Can you work these out from the model? Positions are in its coordinate system, mm. Face numbers are marked on the shaded views. A direction names the side the tool comes from. Round coordinates to 2 decimals unless told otherwise and drop trailing zeros. Loops run counter-clockwise (first coordinate to the right, second up) from the corner with the lowest first, then second, coordinate; pieces in that order, holes last. Notation, with made-up numbers: (79.25, -4.75) -> (102.25, -4.75) arc R26 ccw to (102.25, 32.25) -> close; hole circle Ø2 at (35.5, -18). An arc over 180 degrees is marked (long way). Answer as a JSON object with one key per item and string values.
```python
from build123d import *

# Parameters (mm, degrees)
SKETCH1_W                        = 25.4
SKETCH1_H                        = 141.2875
EXTRUDE1_DEPTH                   = 6.35
CUT_EXTRUDE1_REACH               = 74.891
SKETCH2_R                        = 9.525
CUT_EXTRUDE2_REACH               = 74.891
CHAMFER1_SIZE                    = 15.875
CHAMFER1_SIZE2                   = 4.25369343
F_21_64_0_32813_DIAMETER_HOLE1_D = 8.334502
F_1_4_20_TAPPED_HOLE1_D          = 5.1054
F_10_32_TAPPED_HOLE1_D           = 4.0386
F_10_32_TAPPED_HOLE1_DEPTH       = 13.716
F_10_32_TAPPED_HOLE1_TIP         = 1.213317848
FILLET1_R                        = 6.35
CHAMFER2_SIZE                    = 3.175


with BuildPart() as part:
    # Sketch1 → Extrude1 (new, symmetric)
    with BuildSketch(Plane.XY):
        Rectangle(SKETCH1_W, SKETCH1_H)
    extrude(amount=EXTRUDE1_DEPTH, both=True)

    # Sketch2 → Cut-Extrude1 (cut, up to next)
    with BuildSketch(Plane.XY.offset(6.35), mode=Mode.PRIVATE) as cut_extrude1_sk1:
        with Locations((0, 56.35625)):
            Circle(SKETCH2_R)
    cut_extrude1_tool1 = extrude(cut_extrude1_sk1.sketch, amount=-CUT_EXTRUDE1_REACH, mode=Mode.PRIVATE) & part.part
    add(cut_extrude1_tool1.solids().sort_by_distance((0, 56.35625, 6.35))[0], mode=Mode.SUBTRACT)

    # Sketch3 → Cut-Extrude2 (cut, up to next)
    with BuildSketch(Plane.XY.offset(6.35), mode=Mode.PRIVATE) as cut_extrude2_sk1:
        with BuildLine():
            Line((6.35, -57.94375), (0.79375, -57.94375))
            ThreePointArc((0.79375, -57.94375), (0.232483992, -57.711266008), (0, -57.15))
            Line((0, -57.15), (0, -19.84375))
            ThreePointArc((0, -19.84375), (1.859871939, -15.353621939), (6.35, -13.49375))
            Line((6.35, -13.49375), (12.7, -13.49375))
            Line((12.7, -13.49375), (12.7, -70.64375))
            Line((12.7, -70.64375), (6.35, -70.64375))
            Line((6.35, -70.64375), (6.35, -57.94375))
        make_face()
    cut_extrude2_tool1 = extrude(cut_extrude2_sk1.sketch, amount=-CUT_EXTRUDE2_REACH, mode=Mode.PRIVATE) & part.part
    add(cut_extrude2_tool1.solids().sort_by_distance((6.820727, -39.618194, 6.35))[0], mode=Mode.SUBTRACT)

    # Chamfer1
    chamfer1_edges = [part.edges().sort_by_distance(p)[0] for p in [
        (12.7, 70.64375, 0),
    ]]
    chamfer1_side = [part.faces().sort_by_distance(p)[0] for p in [
        (12.7, 28.575, 0),
    ]]
    chamfer(chamfer1_edges, length=CHAMFER1_SIZE, length2=CHAMFER1_SIZE2, reference=chamfer1_side[0])

    # 21/64 (0.32813) Diameter Hole1 (through all)
    with Locations(Plane.XY.offset(6.35)):
        with Locations((6.35, -3.96875)):
            Hole(F_21_64_0_32813_DIAMETER_HOLE1_D / 2)

    # 1/4-20 Tapped Hole1 (through all)
    with Locations(Plane.XY.offset(6.35)):
        with Locations((0, -64.29375)):
            Hole(F_1_4_20_TAPPED_HOLE1_D / 2)

    # #10-32 Tapped Hole1
    with Locations(Plane.ZY.offset(12.7)):
        with Locations((0, -50.00625), (0, -37.30625)):
            Hole(F_10_32_TAPPED_HOLE1_D / 2, depth=F_10_32_TAPPED_HOLE1_DEPTH)
            with Locations((0, 0, -(F_10_32_TAPPED_HOLE1_DEPTH + F_10_32_TAPPED_HOLE1_TIP / 2))):  # 118° drill point
                Cone(0, F_10_32_TAPPED_HOLE1_D / 2, F_10_32_TAPPED_HOLE1_TIP, mode=Mode.SUBTRACT)

    # Fillet1
    fillet1_edges = [part.edges().sort_by_distance(p)[0] for p in [
        (12.7, -13.49375, 0),
    ]]
    fillet(fillet1_edges, radius=FILLET1_R - 0.0001)  # a hair under: the kernel refuses the full size

    # Chamfer2
    chamfer2_edges = [part.edges().sort_by_distance(p)[0] for p in [
        (-12.7, -70.64375, 0),
    ]]
    chamfer(chamfer2_edges, length=CHAMFER2_SIZE)


solid = part.part
```
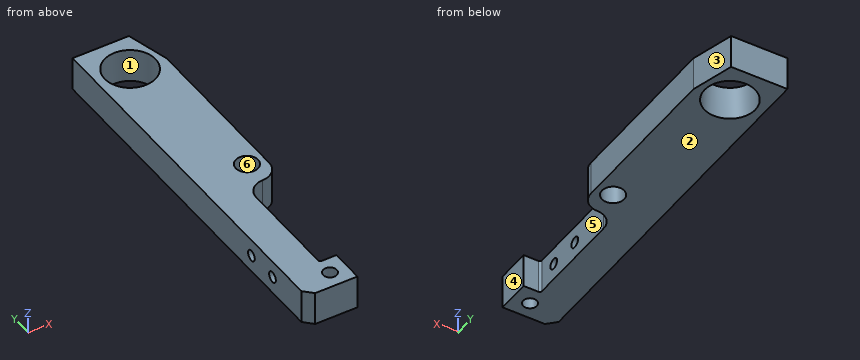
Q1. I want a section at B-B, the plane x = -4.75. Write out the boundary of the cut face in (y, z), then the cut area to 3 significant figures.
Determined:
{"outline": "(-70.64, -6.35) -> (48.1, -6.35) -> (48.1, 6.35) -> (-70.64, 6.35) -> close; (64.61, -6.35) -> (70.64, -6.35) -> (70.64, 6.35) -> (64.61, 6.35) -> close; hole circle Ø4.04 at (-50.01, 0); hole circle Ø4.04 at (-37.31, 0)", "area": "1,560 mm²"}
Q2. On a 3-axis mill with a long thin cutter (end or side, diameter ignored), from which of +Z, -Z, +X, -X, +Y, -Y can I reach the whole of each face in a straight line? I mean the marked faces 4, 5 and 6. Say none if no direction works.
Determined:
{"face 4": "+Z, -Z, +X, -Y", "face 5": "+Z, -Z, +X", "face 6": "+Z, -Z"}
Q3. I want a section at C-C, the plane y = 49. Write out the boundary of the cut face in (x, z).
Determined:
{"outline": "(-12.7, -6.35) -> (-6.05, -6.35) -> (-6.05, 6.35) -> (-12.7, 6.35) -> close; (6.05, -6.35) -> (12.7, -6.35) -> (12.7, 6.35) -> (6.05, 6.35) -> close"}
Q4. If I drill on L1, parallel to Y at x = -3.25, z = 0; L2, parallel to Y at x = 5.25, z = 3.25; L3, parallel to Y at x = -10.75, z = 1, over which ranges is the centre line in solid material (lowest first)? Write a range as [from, to].
Determined:
{"L1": "[-70.64, -52.03], [-47.99, -39.33], [-35.29, 47.4], [65.31, 70.64]", "L2": "[-70.64, -57.94], [-13.59, -7.99], [0.05, 48.41], [64.3, 70.64]", "L3": "[-69.42, -51.76], [-48.25, -39.06], [-35.55, 70.64]"}
Q5. We'd pull the mould along X, two halves only. Please class the marked faces 1, 2 and 3: pulls with the +X half, pulls with the -X half, needs draft (parallel to the pull), parting line crosses it, or undercut.
Determined:
{"face 1": "undercut", "face 2": "needs draft", "face 3": "pulls with the +X half"}
Q6. I'm going to push flat-ended pins straight in: pin 1 (5.5 mm diameter, centred on y = -37.31, z = 0, fed in from +X); pin 2 (4 mm diameter, centred on y = -62, z = -2, fed in from +X). Where does each tip first touch, or does it pass through?
Determined:
{"pin 1": "x = 0", "pin 2": "x = 6.35"}
Q7. I want a section at A-A, the plane z = -0.75. Give the number of separate pieces and of enclosed holes in the cut face, then the cut area to 3 significant figures.
Determined:
{"separate pieces": "3", "enclosed holes": "3", "area": "2,450 mm²"}
